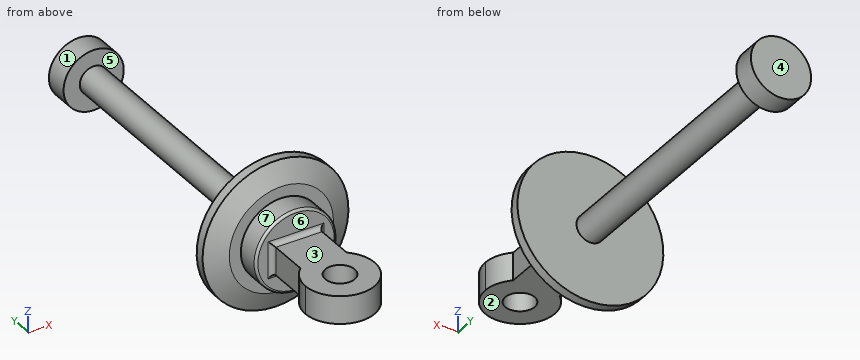
```python
from build123d import *
from build123d.topology import SkipClean

# Parameters (mm, degrees)
BOSS_EXTRUDE1_DEPTH = 6
SKETCH2_R           = 6.35
CUT_EXTRUDE1_DEPTH  = 36.623026261
CUT_EXTRUDE2_DEPTH  = 36.623026261
SKETCH4_R           = 17.5
BOSS_EXTRUDE2_DEPTH = 10
FILLET3_R           = 1
FILLET4_R           = 2
SKETCH6_R           = 6
BOSS_EXTRUDE3_DEPTH = 130
SKETCH7_R           = 13
BOSS_EXTRUDE4_DEPTH = 10


with BuildPart() as part:
    # Sketch1 → Boss-Extrude1 (new, symmetric)
    with BuildSketch(Plane.XY):
        with BuildLine():
            Line((-15, 15), (15, 15))
            Line((15, 15), (15, -15))
            ThreePointArc((15, -15), (0, -30), (-15, -15))
            Line((-15, -15), (-15, 15))
        make_face()
    extrude(amount=BOSS_EXTRUDE1_DEPTH, both=True)

    # Sketch2 → Cut-Extrude1 (cut, through all)
    with BuildSketch(Plane.XY.offset(6)):
        with Locations((0, -15)):
            Circle(SKETCH2_R)
    extrude(amount=-CUT_EXTRUDE1_DEPTH, mode=Mode.SUBTRACT)

    # Sketch3 → Cut-Extrude2 (cut, through all)
    with SkipClean():  # the faces are left unmerged after this step: merging them gives an invalid solid
        with BuildSketch(Plane.XY.offset(6)):
            with BuildLine():
                Line((-10, -3.819660113), (-10, 15))
                Line((-10, 15), (-15, 15))
                Line((-15, 15), (-15, -15))
                ThreePointArc((-15, -15), (-13.693063938, -8.876275643), (-10, -3.819660113))
            make_face()
            with BuildLine():
                Line((15, 15), (15, -15))
                ThreePointArc((15, -15), (13.693063938, -8.876275643), (10, -3.819660113))
                Line((10, -3.819660113), (10, 15))
                Line((10, 15), (15, 15))
            make_face()
        extrude(amount=-CUT_EXTRUDE2_DEPTH, mode=Mode.SUBTRACT)

    # Sketch4 → Boss-Extrude2 (add)
    with BuildSketch(Plane(origin=(0, 15, 0), x_dir=(1, 0, 0), z_dir=(0, 1, 0))):
        with Locations(Location((0, 0, 0), (0, 0, 270))):
            Circle(SKETCH4_R)
    extrude(amount=BOSS_EXTRUDE2_DEPTH)

    # Fillet3
    fillet3_edges = [part.edges().sort_by_distance(p)[0] for p in [
        (0, 15, -17.5),
    ]]
    fillet(fillet3_edges, radius=FILLET3_R)

    # Fillet4
    fillet4_edges = [part.edges().sort_by_distance(p)[0] for p in [
        (-10, 15, 0),
        (0, 15, -6),
        (0, 15, 6),
        (10, 15, 0),
    ]]
    fillet(fillet4_edges, radius=FILLET4_R)

    # Sketch5 → Revolve1 (revolve)
    with BuildSketch(Plane(origin=(0, 0, 0), x_dir=(0, 0, -1), z_dir=(1, 0, 0)), mode=Mode.PRIVATE) as revolve1_sk:
        Polygon((0, 25), (-22.5, 25), (-31.5, 29), (-31.5, 33), (0, 33), align=None)
    revolve(revolve1_sk.sketch.rotate(Axis((0, 0, 0), (0, 1, 0)), 180), axis=Axis((0, 0, 0), (0, 1, 0)))

    # Sketch6 → Boss-Extrude3 (add)
    with BuildSketch(Plane(origin=(0, 33, 0), x_dir=(1, 0, 0), z_dir=(0, 1, 0))):
        with Locations(Location((0, 0, 0), (0, 0, 90))):
            Circle(SKETCH6_R)
    extrude(amount=BOSS_EXTRUDE3_DEPTH)

    # Sketch7 → Boss-Extrude4 (add)
    with BuildSketch(Plane(origin=(0, 163, 0), x_dir=(1, 0, 0), z_dir=(0, 1, 0))):
        with Locations(Location((0, 0, 0), (0, 0, 270))):
            Circle(SKETCH7_R)
    extrude(amount=-BOSS_EXTRUDE4_DEPTH)


solid = part.part
```
Input: part model. Units: mm. Frame: model coordinates. Face numbers are marked on the shaded views. A direction names the side the tool comes from. Round coordinates to 2 decimals unless told otherwise and drop trailing zeros. Order: outer loops, then holes, each group sorted by start corner. A loop starts at its lowest first (then second) coordinate and runs counter-clockwise, first axis right, second up. Notation, with made-up numbers: (-26, 60.25) - (14, 60.25) arc R15 ccw to (14, 77.25) - close; hole circle Ø4 at (-29, 0.25). An arc over 180 degrees is marked (long way). One line per question, with ' | ' between items. Start each with the question number.
1) Cut plane C-C, the plane y = -1. Return the cut outline in (x, z).
2) Cut plane D-D, the plane y = 122. Return the cut outline in (x, z), then the cut area to 3 significant figures.
3) Ray query, probe 1 along Y at (x, z) = (0, 2.75); probe 2 along Y at (x, z) = (-18.5, -3); probe 3 along Y at (x, z) = (-13.5, -4.5). Return the intervals inside material, ascending.
4) Contact query for flat-ended pins moving along their axis: P1, Ø9, axis at x = -4, y = -3, coming from the -Z side; P2, Ø10, axis at x = 0, y = -15, coming from the -Z side; P3, Ø4, axis at y = 51, z = 2, coming from the -X side; P4, Ø1.5, axis at x = 3.5, y = 20, coming from the +Z side. Output: stop coordinate, or through.
5) Pull-direction query (Y, two-part tool) for the marked faces 4, 5, 6 and 7; classes: +Y half, -Y half, draft (parallel to the pull), parting line (faces both ways), or undercut.
6) Set-up query: the marked faces 1, 2 and 3. Return all of +Z, -Z, +X, -X, +Y, -Y with unobstructed straight access to the full face (end or side cutting, diameter ignored); none if empty.
7) Cut plane B-B, the plane z = 0. Return the cut outline in (x, y), then the cut area to 3 significant figures.
Worked out:
1) outline: (-10, -6) - (10, -6) - (10, 6) - (-10, 6) - close
2) outline: circle Ø12 at (0, 0) | area: 113 mm^2
3) probe 1: y = -30 to -21.35, -8.65 to 163 | probe 2: y = 25 to 33 | probe 3: y = -21.54 to -8.46, 15 to 33
4) P1: stops at z = -6 | P2: passes through | P3: stops at x = -6 | P4: stops at z = 17.28
5) face 4: +Y half | face 5: undercut | face 6: undercut | face 7: draft
6) face 1: +Y | face 2: -Z, +X, -X, -Y | face 3: +Z, +X, -X, -Y
7) outline: (-31.5, 29) - (-22.5, 25) - (-17.5, 25) - (-17.5, 16) arc R1 ccw to (-16.5, 15) - (-12, 15) arc R2 cw to (-10, 13) - (-10, -3.82) arc R15 ccw (long way) to (10, -3.82) - (10, 13) arc R2 cw to (12, 15) - (16.5, 15) arc R1 ccw to (17.5, 16) - (17.5, 25) - (22.5, 25) - (31.5, 29) - (31.5, 33) - (6, 33) - (6, 153) - (13, 153) - (13, 163) - (-13, 163) - (-13, 153) - (-6, 153) - (-6, 33) - (-31.5, 33) - close; hole circle Ø12.7 at (0, -15) | area: 3,420 mm^2
